Geometry check sheet. Reference: the model listing, model coordinates, mm. A direction names the side the tool comes from. Round coordinates to 2 decimals unless told otherwise and drop trailing zeros. Write each loop counter-clockwise with the first axis right and the second up, starting at its lowest first coordinate (ties: lowest second). Pieces come first, ordered by that corner, then holes.
Item 1: Depth check by flat-ended pin: P1, Ø1, axis at y = -19, z = 19.5, coming from the +X side; P2, Ø10, axis at x = -26.5, y = -6.5, coming from the +Z side; P3, Ø2, axis at y = -13.5, z = -12.5, coming from the +X side. Enter the tip coordinate at first touch or a pass-through.
Item 2: Cross-section at A-A (y = -8.5). Enter the section's corners in (x, z), then the cut area to 3 significant figures.
Item 3: Cross-section at B-B (x = 0). Enter the section's corners in (y, z).
Item 4: Draft check along Z on faces 3 (the face through (-42, -13, 3.81)), 4 (the face through (-14, -25.4, -16)), 5 (the face through (-39.741, -12.522, -12.626)), 6 (the face through (-36.885, -12.522, -19.644)). Enter one of: pulls with the +Z half, pulls with the -Z half, needs draft (parallel to the pull), parting line crosses it, or undercut.
Item 5: Cross-section at C-C (x = 20). Enter the section's corners in (y, z).
Item 6: Access from +Z, -Z, +X, -X, +Y, -Y to the whole of each face (thin tool, end or side, straight path). Record for faces 1 (the face through (-15.12, -12.52, -11.59)), 2 (the face through (-37.367, -12.522, -7.435)).
Item 7: Cross-section at D-D (z = -22.5). Enter the section's corners in (x, y), then the cut area to 3 significant figures.
Item 8: Scan lines: probe 1 along Z at (x, y) = (0, -18); probe 2 along Z at (x, y) = (-10.5, -15.25); probe 3 along X at (y, z) = (-10.75, 7). Record each from-to range of solid material in increasing order.
from build123d import *

# Parameters (mm, degrees)
F0_R     = 19.05
F1_DEPTH = 25.4


with BuildPart() as f1:
    # F0 (on Front) → F1 (new body)
    with BuildSketch(Plane.XZ):
        with BuildLine():
            ThreePointArc((-33.535455, -18.082679), (9.324944, -36.941243), (38.1, 0))
            ThreePointArc((38.1, 0), (1.907392, 38.052225), (-37.909021, 3.81))
            ThreePointArc((-37.909021, 3.81), (-38.1, 0), (-37.909021, -3.81))
            ThreePointArc((-37.909021, -3.81), (-37.357291, -7.486173), (-36.449937, -11.091082))
            ThreePointArc((-36.449937, -11.091082), (-35.166879, -14.659489), (-33.535455, -18.082679))
        make_face()
        Circle(F0_R, mode=Mode.SUBTRACT)
        with BuildLine():
            ThreePointArc((-37.909021, -3.81), (-38.1, 0), (-37.909021, 3.81))
            Line((-37.909021, 3.81), (-45.281142, 3.81))
            ThreePointArc((-45.281142, 3.81), (-45.819958, 3.586815), (-46.043142, 3.048))
            Line((-46.043142, 3.048), (-46.043142, 0))
            Line((-46.043142, 0), (-46.043142, -3.048))
            ThreePointArc((-46.043142, -3.048), (-45.815414, -3.586136), (-45.275021, -3.808454))
            Line((-45.275021, -3.808454), (-37.909021, -3.81))
        make_face()
        with BuildLine():
            Line((-40.141169, -21.162974), (-33.535455, -18.082679))
            ThreePointArc((-33.535455, -18.082679), (-35.166879, -14.659489), (-36.449937, -11.091082))
            Line((-36.449937, -11.091082), (-43.1258, -14.204088))
            ThreePointArc((-43.1258, -14.204088), (-43.519811, -14.634075), (-43.494372, -15.216729))
            Line((-43.494372, -15.216729), (-42.228101, -17.932256))
            Line((-42.228101, -17.932256), (-40.93996, -20.694683))
            ThreePointArc((-40.93996, -20.694683), (-40.663444, -21.138431), (-40.141169, -21.162974))
        make_face()
    extrude(amount=F1_DEPTH)


solid = f1.part
Resolved:
1. P1: stops at x = 33.02
1. P2: stops at z = 31.45
1. P3: stops at x = 36.32
2. outline: (-46.04, -3.05) arc R0.77 ccw to (-45.28, -3.81) - (-37.91, -3.81) arc R38.1 ccw to (-36.45, -11.09) - (-43.13, -14.2) arc R0.76 ccw to (-43.49, -15.22) - (-40.94, -20.69) arc R0.56 ccw to (-40.14, -21.16) - (-33.54, -18.08) arc R38.1 ccw (long way) to (-37.91, 3.81) - (-45.28, 3.81) arc R0.76 ccw to (-46.04, 3.05) - close; hole circle Ø38.1 at (0, 0)
2. area: 3,540 mm2
3. outline: (-25.4, -38.1) - (0, -38.1) - (0, -19.05) - (-25.4, -19.05) - close; (-25.4, 19.05) - (0, 19.05) - (0, 38.1) - (-25.4, 38.1) - close
4. face 3: pulls with the +Z half
4. face 4: needs draft
4. face 5: undercut
4. face 6: pulls with the -Z half
5. outline: (-25.4, -32.43) - (0, -32.43) - (0, 32.43) - (-25.4, 32.43) - close
6. face 1: +Y, -Y
6. face 2: -X, +Y, -Y
7. outline: (-30.75, -25.4) - (30.75, -25.4) - (30.75, 0) - (-30.75, 0) - close
7. area: 1,560 mm2
8. probe 1: z = -38.1 to -19.05, 19.05 to 38.1
8. probe 2: z = -36.62 to -15.9, 15.9 to 36.62
8. probe 3: x = -37.45 to -17.72, 17.72 to 37.45
